Autodesk Inventor part; units mm, degrees
ref_plane "Work Plane1" through (0, 12, 0) normal (0, 1, 0) x (-1, 0, 0)
ref_plane "Work Plane2" through (0, 7, 0) normal (0, 1, 0) x (-1, 0, 0)
ref_plane "YZ Plane" through (0, 0, 0) normal (1, 0, 0) x (0, 1, 0)
sketch "Sketch1" plane through (0, 0, 0) normal (0, 0, 1) x (1, 0, 0)
  circle A0 centre (0, 0) radius 12
  dimension "d0" = 24
extrude "Extrusion1" add sketch "Sketch1" against normal blind 10
sketch "Sketch2" plane through (0, 0, 0) normal (0, 0, 1) x (1, 0, 0)
  circle A0 centre (0, 0) radius 7
  dimension "d3" = 14
extrude "Extrusion2" add sketch "Sketch2" along normal blind 15
fillet "Fillet1" radius 1 3 edges at (-7, 0, 0) (-12, 0, 0) (-12, 0, -10)
ref_plane "Work Plane1" through (0, 12, 0) normal (0, 1, 0) x (-1, 0, 0)
sketch "Sketch4" plane through (0, 12, 0) normal (0, 1, 0) x (-1, 0, 0)
  line L0 (11, -10) -> (-11, -10)
  point P0 (0, 0)
  point P1 (0, -4)
  dimension "d15" = 6
hole "Hole2" at (0, 12, -4) direction (0, -1, 0) diameter 5 depth 8
pattern_circular "Circular Pattern1" count 6 over 360 about axis through (0, 0, -9) along (0, 0, -1) of "Hole2"
ref_plane "Work Plane2" through (0, 7, 0) normal (0, 1, 0) x (-1, 0, 0)
sketch "Sketch5" plane through (0, 7, 0) normal (0, 1, 0) x (-1, 0, 0)
  line L0 (7, 15) -> (-7, 15)
  line L1 (2.3094, -4.9574) -> (2.3094, -3.0426)
  arc A0 (2.3094, -3.0426) -> (-2.3094, -3.0426) centre (0, -4) ccw
  line L2 (-2.3094, -3.0426) -> (-2.3094, -4.9574)
  arc A1 (-2.3094, -4.9574) -> (2.3094, -4.9574) centre (0, -4) ccw
  point P0 (0, 0)
  point P1 (0, 4)
  point P2 (0, -6.5)
  point P3 (0, -1.5)
  point P4 (0, -3.5)
  point P5 (0, -8.5)
  point P6 (0, -2.5)
  point P7 (0, -7.5)
  dimension "d27" = 11
hole "Hole3" at (0, 7, 4) direction (0, -1, 0) diameter 2.459 end through all
sketch "Sketch6" plane through (0, 0, 15) normal (0, 0, 1) x (1, 0, 0)
  circle A0 centre (0, 0) radius 7
hole "Hole4" at (0, 0, 15) direction (0, 0, -1) diameter 6 depth 25
properties part number "22.4" material "Lead"
Input: part model. Units: mm. Frame: model coordinates. A direction names the side the tool comes from. Give positions to 0.01 mm unless a question says otherwise; leave off trailing zeros. Order: outer loops, then holes, each group sorted by start corner. A loop starts at its lowest first (then second) coordinate and runs counter-clockwise, first axis right, second up.
Q1. Contact query for flat-ended pins moving along their axis: pin 1 Ø8 at (x, z) = (0, -4) entering from -Y; pin 2 Ø2 at (x, z) = (0, 4) entering from +Y; pin 3 Ø2.5 at (x, z) = (0.5, -4.5) entering from +Y; pin 4 Ø3 at (x, y) = (-9, 3) entering from +Z. Output: stop coordinate, or through.
Checked values:
pin 1: stops at y = -12
pin 2: passes through
pin 3: stops at y = 4
pin 4: stops at z = 0
Q2. Draft query along Z for faces 4 (the cylindrical face through (-0.9, -2.86, 2.32)), 5 (the flat face through (3.448, 2.028, -4.035)), 6 (the flat face through (-2, -8, 0)). Return one class per face: +Z half, -Z half, draft (parallel to the pull), parting line (faces both ways), or undercut.
Checked values:
face 4: draft
face 5: undercut
face 6: +Z half
Q3. Ray query, probe 1 along Z at (x, y) = (0, 5.5); probe 2 along Y at (x, z) = (-5, -2.25); probe 3 along Y at (x, z) = (7.5, -4.25). Return the intervals inside material, ascending.
Checked values:
probe 1: z = -10 to -6.5, -1.5 to 2.77, 5.23 to 15
probe 2: y = -10.91 to -4.95, -0.83 to 0.83, 4.95 to 10.91
probe 3: y = -9.37 to -7.2, -1.46 to 1.46, 7.2 to 9.37
Q4. Section C-C on z = 4. Output: boundary loops of the cut face in (x, y), and give its area (3 significant figures).
Checked values:
outline: (-1.23, -6.89) - (-1.23, -2.74) arc R3 cw to (-1.23, 2.74) - (-1.23, 6.89) arc R7 ccw to start; (1.23, -6.89) arc R7 ccw to (1.23, 6.89) - (1.23, 2.74) arc R3 cw to (1.23, -2.74) - close
area: 106 mm2
Q5. Section A-A on x = 0. State how many separate pieces and enclosed holes the cut face has, and give its area (3 significant figures).
Checked values:
separate pieces: 4
enclosed holes: 0
area: 200 mm2
Q6. Section B-B on z = -4. Output: boundary loops of the cut face in (x, y), and give its area (3 significant figures).
Checked values:
outline: (-11.41, -3.7) - (-5, 0) - (-11.41, 3.7) arc R12 ccw to start; (-8.91, -8.03) arc R12 ccw to (-2.5, -11.74) - (-2.5, -4.33) - close; (-8.91, 8.03) - (-2.5, 4.33) - (-2.5, 11.74) arc R12 ccw to start; (-4.62, 0) - (-2.31, -4) - (2.31, -4) - (4.62, 0) - (2.31, 4) - (-2.31, 4) - close; (2.5, -11.74) arc R12 ccw to (8.91, -8.03) - (2.5, -4.33) - close; (2.5, 4.33) - (8.91, 8.03) arc R12 ccw to (2.5, 11.74) - close; (5, 0) - (11.41, -3.7) arc R12 ccw to (11.41, 3.7) - close; hole circle Ø6 at (0, 0)
area: 187 mm2
Q7. Set-up query: faces 1 (the cylindrical face through (-0.751, 7.944, -1.615)), 2 (the flat face through (-3.48, 1.97, -4.04)), 3 (the cylindrical face through (0.751, -7.944, -1.615)). Return all of +Z, -Z, +X, -X, +Y, -Y with unobstructed straight access to the full face (end or side cutting, diameter ignored); none if empty.
Checked values:
face 1: +Y
face 2: none
face 3: -Y
